The drawing under review shows one solid part. Ordinate dimensions are in mm from its lowest x, y, z. A direction names the side the tool comes from. Round coordinates to 2 decimals unless told otherwise and drop trailing zeros. Order: outer loops, then holes, each group sorted by start corner. A loop starts at its lowest first (then second) coordinate and runs counter-clockwise, first axis right, second up. Notation, with made-up numbers: (-36.75, 27.25) - (-2.75, 27.25) arc R35 ccw to (-2.75, 65.25) - close; hole circle Ø7 at (-26.5, 71). An arc over 180 degrees is marked (long way). One line per question, with ' | ' between items.
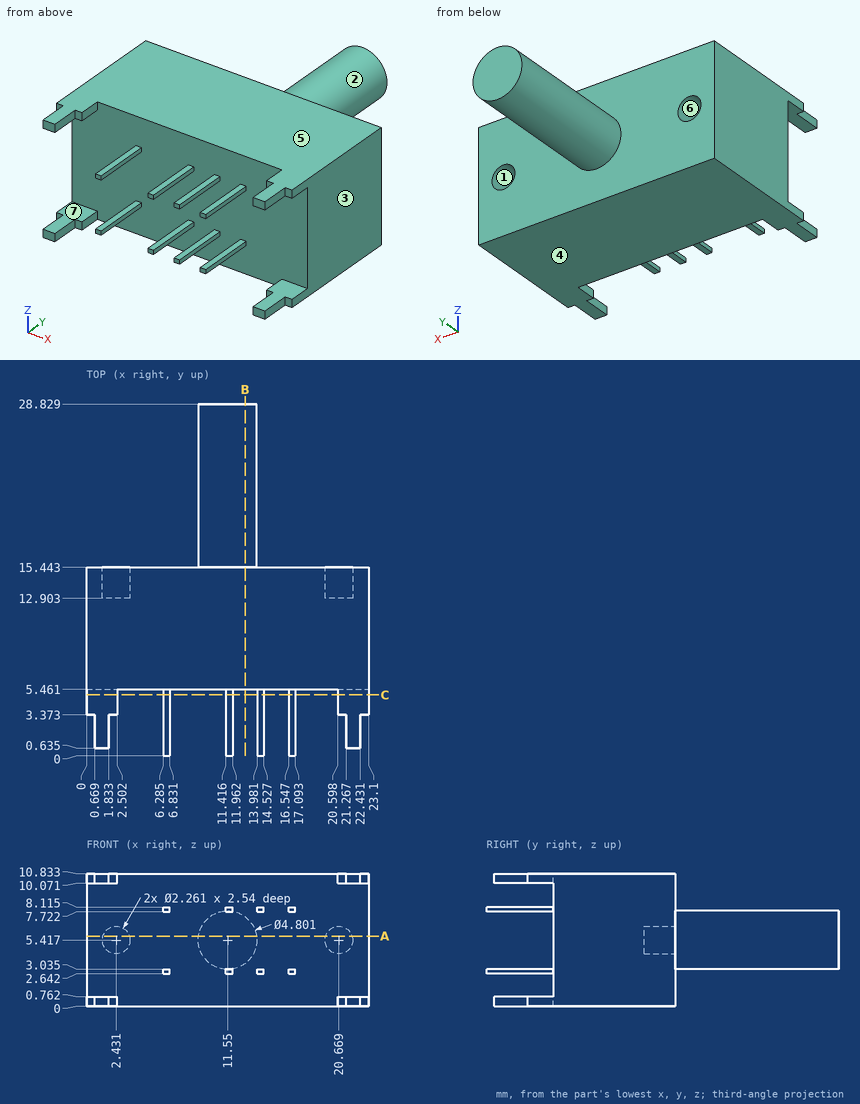
(1) Insertion check: pin 1 (1.5 mm diameter, centred on x = 20, y = 16.5, fed in from -Z); pin 2 (0.8 mm diameter, centred on y = 2, z = 10.5, fed in from -X); pin 3 (3 mm diameter, centred on x = 20.67, z = 5.42, fed in from +Y); pin 4 (2 mm diameter, centred on x = 8, z = 9, fed in from -Y). Each pin has a flat end and moves straight along its axis. Give the tip position at first contact, or say it passes through.
Output values:
pin 1: through | pin 2: x = 0.67 | pin 3: y = 15.44 | pin 4: y = 5.46
(2) For the marked faces 5, 6 and 7, list the 3-axis set-ups (+Z, -Z, +X, -X, +Y, -Y) from which the entire face can be reached by the end or side of a thin tool; tool diameter is ignored.
Output values:
face 5: +Z, +X, -X, +Y, -Y | face 6: +Y | face 7: +X, -X, -Y
(3) Mouldability with a two-part tool opening along Z and no side actions: class the marked faces 1, 2, 3 and 4 as released by +Z, released by -Z, zero draft, split by the parting line, or undercut.
Output values:
face 1: undercut | face 2: split by the parting line | face 3: zero draft | face 4: released by -Z
(4) For probe 1 along Z at (x, y) = (20.75, 15) (1 decimal); probe 2 along Y at (x, z) = (18.75, 3.25); probe 3 along Z at (x, y) = (11.75, 23.75) (1 decimal), list the stretches that pass through material, from the lowest coordinate up. Write a range as [from, to].
Output values:
probe 1: [0, 4.3], [6.5, 10.8] | probe 2: [5.46, 15.44] | probe 3: [3, 7.8]
(5) We need section B-B on x = 13. State the section outline as (y, z) points.
Output values:
outline: (5.46, 0) - (15.44, 0) - (15.44, 3.5) - (28.83, 3.5) - (28.83, 7.33) - (15.44, 7.33) - (15.44, 10.83) - (5.46, 10.83) - close
(6) We need section C-C on y = 5. Give the number of separate pieces and of enclosed holes in the cut face.
Output values:
separate pieces: 12 | enclosed holes: 0
(7) We need section A-A on z = 5.75. State the section outline as (x, y) points, plus the area to 3 significant figures.
Output values:
outline: (0, 5.46) - (23.1, 5.46) - (23.1, 15.44) - (21.75, 15.44) - (21.75, 12.9) - (19.59, 12.9) - (19.59, 15.44) - (13.93, 15.44) - (13.93, 28.83) - (9.17, 28.83) - (9.17, 15.44) - (3.51, 15.44) - (3.51, 12.9) - (1.35, 12.9) - (1.35, 15.44) - (0, 15.44) - close | area: 283 mm^2
